```python
from build123d import *

# Parameters (mm, degrees)
BOSS_EXTRU_1_DEPTH      = 6.35
ENL_V_MAT_EXTRU_2_DEPTH = 232.027391955
ESQUISSE5_R             = 1.5
ENL_V_MAT_EXTRU_3_DEPTH = 5
ESQUISSE7_R             = 1.5
ENL_V_MAT_EXTRU_4_DEPTH = 5
ESQUISSE8_R             = 1.5
ENL_V_MAT_EXTRU_5_DEPTH = 5


with BuildPart() as part:
    # Esquisse2 → Boss.-Extru.1 (new body)
    with BuildSketch(Plane.XY):
        Polygon((-115.470053838, 0), (115.470053838, 0), (0, 200), align=None)
    extrude(amount=BOSS_EXTRU_1_DEPTH)

    # Esquisse4 → Enlèv. mat.-Extru.2 (cut, through all)
    with BuildSketch(Plane.XY.offset(6.35)):
        Polygon((-115.470053838, 0), (-93.470053838, 38.105117767), (-71.470053838, 0), align=None)
        Polygon((115.470053838, 0), (71.470053838, 0), (93.470053838, 38.105117767), align=None)
        Polygon((0, 200), (-22, 161.894882233), (22, 161.894882233), align=None)
    extrude(amount=-ENL_V_MAT_EXTRU_2_DEPTH, mode=Mode.SUBTRACT)

    # Esquisse5 → Enlèv. mat.-Extru.3 (cut)
    with BuildSketch(Plane(origin=(-53.602540378, -30.947441117, 0), x_dir=(0, 0, 1), z_dir=(-0.8660254037844389, -0.49999999999999983, 0))):
        with Locations(Location((3.175, 57.735026919, 0), (0, 0, 270))):
            Circle(ESQUISSE5_R)
    extrude(amount=-ENL_V_MAT_EXTRU_3_DEPTH, mode=Mode.SUBTRACT)

    # Esquisse7 → Enlèv. mat.-Extru.4 (cut)
    with BuildSketch(Plane(origin=(0, 161.894882233, 0), x_dir=(1, 0, 0), z_dir=(0, 1, 0))):
        with Locations(Location((0, -3.175, 0), (0, 0, 270))):
            Circle(ESQUISSE7_R)
    extrude(amount=-ENL_V_MAT_EXTRU_4_DEPTH, mode=Mode.SUBTRACT)

    # Esquisse8 → Enlèv. mat.-Extru.5 (cut)
    with BuildSketch(Plane(origin=(53.602540378, -30.947441117, 0), x_dir=(0, 0, -1), z_dir=(0.8660254037844383, -0.5000000000000009, 0))):
        with Locations(Location((-3.175, 57.735026919, 0), (0, 0, 90))):
            Circle(ESQUISSE8_R)
    extrude(amount=-ENL_V_MAT_EXTRU_5_DEPTH, mode=Mode.SUBTRACT)


solid = part.part
```
Input: part model. Units: mm. Frame: model coordinates. Give positions to 0.01 mm unless a question says otherwise; leave off trailing zeros. Loops run counter-clockwise (first coordinate to the right, second up) from the corner with the lowest first, then second, coordinate; pieces in that order, holes last.
1) Mould query, pull axis Z, two halves, no side actions, for faces 1 (the flat face through (-1, 64, 0)), 2 (the flat face through (-57.235, 100.867, 3.131)), 3 (the cylindrical face through (-79.62, 19.05, 3.63)). Classes: released by +Z, released by -Z, zero draft, split by the parting line, or undercut.
A:
face 1: released by -Z
face 2: zero draft
face 3: undercut
2) Contact query for flat-ended pins moving along their axis: pin 1 (3.5 mm diameter, centred on x = 0, z = 3.175, fed in from -Y); pin 2 (1.5 mm diameter, centred on y = 92, z = 2, fed in from -X); pin 3 (3 mm diameter, centred on y = 41.5, z = 4, fed in from +X); pin 4 (3 mm diameter, centred on y = 130.5, z = 2.5, fed in from -X). Output: stop coordinate, or through.
A:
pin 1: stops at y = 0
pin 2: stops at x = -62.79
pin 3: stops at x = 92.38
pin 4: stops at x = -40.99
3) Line query: L1, parallel to X at y = 90, z = 2.5; L2, parallel to Y at x = -32, z = 1.25; L3, parallel to X at y = 39.5, z = 4.75. Output: solid intervals per line, ascending.
A:
L1: x = -63.51 to 63.51
L2: y = 0 to 144.57
L3: x = -92.66 to 92.66
4) Section query A-A on y = 28.5. Return the cut outline in (x, z).
A:
outline: (-87.92, 0) - (87.92, 0) - (87.92, 6.35) - (-87.92, 6.35) - close
5) Section query B-B on x = -47.5. Return the cut outline in (y, z).
A:
outline: (0, 0) - (117.73, 0) - (117.73, 6.35) - (0, 6.35) - close
